Here's how the part is built. I have some questions about the finished solid (model axes, mm). Face numbers are marked on the shaded views. A direction names the side the tool comes from. Round coordinates to 2 decimals unless told otherwise and drop trailing zeros. Write each loop counter-clockwise with the first axis right and the second up, starting at its lowest first coordinate (ties: lowest second). Pieces come first, ordered by that corner, then holes. Notation, with made-up numbers: (22, 35) - (28, 35) arc R21 ccw to (28, 46) - close; hole circle Ø10 at (30.25, 55.5). An arc over 180 degrees is marked (long way). One line per item, written item: value. Start each with the question number.
Item 1: If I drill on line 1 (X direction, y = -6.5, z = 9.5); line 2 (Z direction, x = -5.7, y = -1.27) (3 decimals); line 3 (X direction, y = 4, z = 23), over which ranges is the centre line in solid material (lowest first)?
Item 2: For the marked faces 1, 2, 3 and 4, which set-ups out of +Z, -Z, +X, -X, +Y, -Y let a thin tool reach every point of the face, with its end or its side?
Item 3: Imagine slicing it at B-B, the plane y = -10.5. Please give me the cut outline in (x, z) (3 decimals).
Item 4: Imagine slicing it at D-D, the plane y = -17. Please give me the cut outline in (x, z) (3 decimals).
Item 5: Thinking about a two-plate mould opening in Y: for the marked faces 5, 6, 7 and 8, which applies, released by +Y, released by -Y, zero draft, split by the parting line, or undercut?
Item 6: Imagine slicing it at C-C, the plane x = -14. Please give me the cut outline in (y, z).
Item 7: Imagine slicing it at A-A, the plane x = 0.5. Please give me the cut outline in (y, z) (3 decimals).
Item 8: For P1, Ø0.8, axis at x = 6.5, z = 14, coming from the +Y side; P2, Ø1.4, axis at x = -0.5, z = 10.5, coming from the -Y side; P3, Ø12, axis at y = -1.5, z = 19.5, coming from the +X side, each with a flat end and sliding along its axis, tell me the tip position at first contact or that it passes through.
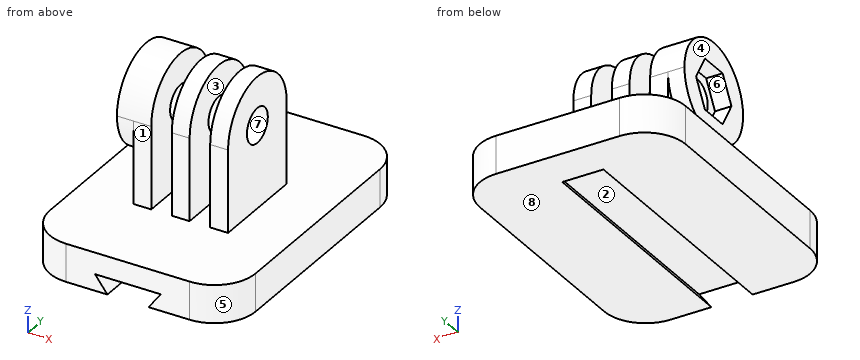
```python
from build123d import *

# Parameters (mm, degrees)
F0_W      = 31.75
F0_H      = 44.45
F1_DEPTH  = 5.842
F3_DEPTH  = 38.1
F4_R      = 2.667
F5_DEPTH  = 9.8425
F6_W      = 2.54
F6_H      = 7.4803
F6_H_2    = 12.7
F6_W_2    = 3.175
F6_H_3    = 5.2197
F7_DEPTH  = 25.4
F9_DEPTH  = 2.54
F10_R     = 6.35
F11_R     = 2.667
F12_DEPTH = 2.54


with BuildPart() as f1:
    # F0 (on Top) → F1 (new body)
    with BuildSketch(Plane.XY):
        Rectangle(F0_W, F0_H)
    extrude(amount=F1_DEPTH)

    # F2 (on face) → F3 (cut)
    with BuildSketch(Plane.XZ.offset(22.225)):
        Polygon((5.08, 2.54), (0, 2.54), (-5.08, 2.54), (-3.175, 0), (3.175, 0), align=None)
    extrude(amount=-F3_DEPTH, mode=Mode.SUBTRACT)

    # F4 (on Right) → F5 (join, symmetric)
    with BuildSketch(Plane.YZ):
        with BuildLine():
            Line((-8.7503, 18.542), (-8.7503, 5.842))
            Line((-8.7503, 5.842), (6.2103, 5.842))
            Line((6.2103, 5.842), (6.2103, 18.542))
            ThreePointArc((6.2103, 18.542), (-1.27, 26.0223), (-8.7503, 18.542))
        make_face()
        with Locations((-1.27, 18.542)):
            Circle(F4_R, mode=Mode.SUBTRACT)
    extrude(amount=F5_DEPTH, both=True)

    # F6 (on face) → F7 (cut)
    with BuildSketch(Plane.XZ.offset(8.7503)):
        with Locations((8.5725, 22.28215)):
            Rectangle(F6_W, F6_H)
        with Locations((8.5725, 12.192)):
            Rectangle(F6_W, F6_H_2)
        with Locations((2.9591, 22.28215)):
            Rectangle(F6_W_2, F6_H)
        with Locations((2.9591, 12.192)):
            Rectangle(F6_W_2, F6_H_2)
        with Locations((-2.9591, 22.28215)):
            Rectangle(F6_W_2, F6_H)
        with Locations((-2.9591, 12.192)):
            Rectangle(F6_W_2, F6_H_2)
        with Locations((-8.5725, 8.45185)):
            Rectangle(F6_W, F6_H_3)
    extrude(amount=-F7_DEPTH, mode=Mode.SUBTRACT)

    # F8 (on face) → F9 (cut)
    with BuildSketch(Plane(origin=(-9.8425, 0, 0), x_dir=(0, -1, 0), z_dir=(-1, 0, 0))):
        with BuildLine():
            ThreePointArc((1.27, 11.0617), (-4.019371, 13.252629), (-6.2103, 18.542))
            Line((-6.2103, 18.542), (-6.2103, 11.0617))
            Line((-6.2103, 11.0617), (1.27, 11.0617))
        make_face()
        with BuildLine():
            ThreePointArc((8.7503, 18.542), (6.559371, 13.252629), (1.27, 11.0617))
            Line((1.27, 11.0617), (8.7503, 11.0617))
            Line((8.7503, 11.0617), (8.7503, 18.542))
        make_face()
    extrude(amount=-F9_DEPTH, mode=Mode.SUBTRACT)

    # F10
    f10_edges = [f1.edges().sort_by_distance(p)[0] for p in [
        (15.875, 22.225, 2.921),
        (-15.875, 22.225, 2.921),
        (-15.875, -22.225, 2.921),
        (15.875, -22.225, 2.921),
    ]]
    fillet(f10_edges, radius=F10_R)

    # F11 (on face) → F12 (cut)
    with BuildSketch(Plane(origin=(-9.8425, 0, 0), x_dir=(0, -1, 0), z_dir=(-1, 0, 0))):
        Polygon((3.528363, 22.4536), (-0.988363, 22.4536), (-3.246727, 18.542), (-0.988363, 14.6304), (3.528363, 14.6304), (5.786727, 18.542), align=None)
        with Locations((1.27, 18.542)):
            Circle(F11_R, mode=Mode.SUBTRACT)
    extrude(amount=-F12_DEPTH, mode=Mode.SUBTRACT)


solid = f1.part
```
Values follow:
1. line 1: x = -7.3 to -4.55, -1.37 to 1.37, 4.55 to 7.3
1. line 2: z = 0 to 15.875, 21.209 to 26.022
1. line 3: x = -9.84 to -4.55, -1.37 to 1.37, 4.55 to 7.3
2. face 1: +Z, +X, -X, -Y
2. face 2: -Y
2. face 3: +Z, +Y, -Y
2. face 4: +Z, -X, +Y, -Y
3. outline: (-15.875, 0) - (-3.175, 0) - (-5.08, 2.54) - (5.08, 2.54) - (3.175, 0) - (15.875, 0) - (15.875, 5.842) - (-15.875, 5.842) - close
4. outline: (-15.775, 0) - (-3.175, 0) - (-5.08, 2.54) - (5.08, 2.54) - (3.175, 0) - (15.775, 0) - (15.775, 5.842) - (-15.775, 5.842) - close
5. face 5: released by -Y
5. face 6: undercut
5. face 7: undercut
5. face 8: zero draft
6. outline: (-20.38, 0) - (20.38, 0) - (20.38, 5.84) - (-20.38, 5.84) - close
7. outline: (-22.225, 2.54) - (15.875, 2.54) - (15.875, 0) - (22.225, 0) - (22.225, 5.842) - (6.21, 5.842) - (6.21, 18.542) arc R7.48 ccw to (-8.75, 18.542) - (-8.75, 5.842) - (-22.225, 5.842) - close; hole circle Ø5.334 at (-1.27, 18.542)
8. P1: stops at y = 6.21
8. P2: stops at y = -8.75
8. P3: stops at x = 7.3
